Check sheet for the modelled part. Datum: model origin and axes. Units: mm. Give positions to 0.01 mm unless a question says otherwise; leave off trailing zeros. Order: outer loops, then holes, each group sorted by start corner. A loop starts at its lowest first (then second) coordinate and runs counter-clockwise, first axis right, second up.
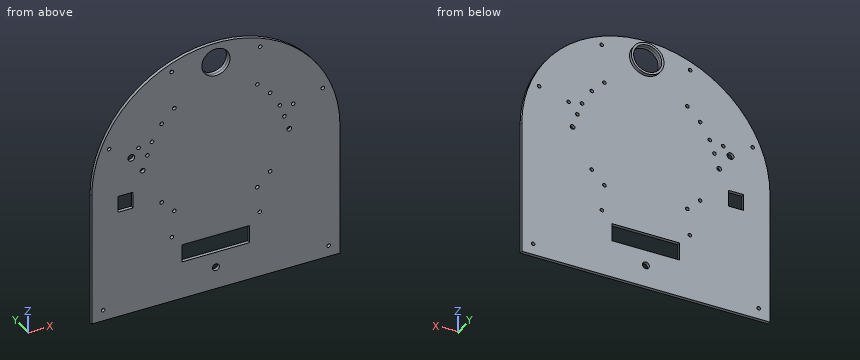
```python
from build123d import *

# Parameters (mm, degrees)
EXTRUDE_START            = -1
EXTRUDE_1_DEPTH          = 3
SKETCH_2_R               = 12.5
CUT_EXTRUDE_1_DEPTH      = 10
SKETCH_3_W               = 220
SKETCH_3_H               = 40
EXTRUDE_2_DEPTH          = 3
CUT_EXTRUDE_2_DEPTH      = 163.815846895
CUT_EXTRUDE_2_DEPTH_BACK = 163.815846895
SKETCH_4_W               = 60
SKETCH_4_H               = 16
SKETCH_5_R               = 1.6
SKETCH_5_R_2             = 2.1
SKETCH_5_R_3             = 3
SKETCH_5_R_4             = 3.1
SKETCH_5_W               = 13.3
SKETCH_5_H               = 14.8
CUT_EXTRUDE_3_DEPTH      = 10
SKETCH_7_R               = 1.6
CUT_EXTRUDE_6_DEPTH      = 162.347451173
SKETCH_8_R               = 1.6
CUT_EXTRUDE_7_DEPTH      = 162.347451173
SHEET_EXTRUDE_1_1_DEPTH  = 3
THICKEN_1_T2             = 2


with BuildPart() as part:
    # 草图1 → 凸台-拉伸1 (new body)
    with BuildSketch(Plane(origin=(0, 0, 0), x_dir=(1, 0, 0), z_dir=(0, 1, 0)).offset(EXTRUDE_START)):
        with BuildLine():
            Line((-110, 0), (-110, 80))
            Line((-110, 80), (110, 80))
            Line((110, 80), (110, 0))
            ThreePointArc((110, 0), (0, -110), (-110, 0))
        make_face()
    extrude(amount=EXTRUDE_1_DEPTH)

    # 草图2 → 切除-拉伸1 (cut)
    with BuildSketch(Plane(origin=(0, 2, 0), x_dir=(1, 0, 0), z_dir=(0, 1, 0))):
        with Locations(Location((0, -92, 0), (0, 0, 270))):
            Circle(SKETCH_2_R)
    extrude(amount=-CUT_EXTRUDE_1_DEPTH, mode=Mode.SUBTRACT)

    # 草图3 → 凸台-拉伸2 (add)
    with BuildSketch(Plane(origin=(0, 2, 0), x_dir=(1, 0, 0), z_dir=(0, 1, 0))):
        with Locations((0, 100)):
            Rectangle(SKETCH_3_W, SKETCH_3_H)
    extrude(amount=-EXTRUDE_2_DEPTH)

    # 草图4 → 切除-拉伸2 (cut, two sides: drawn at the far end of the back side and taken through both)
    with BuildSketch(Plane(origin=(0, 2, 0), x_dir=(1, 0, 0), z_dir=(0, 1, 0)).offset(-CUT_EXTRUDE_2_DEPTH_BACK)):
        with Locations((0, 78)):
            Rectangle(SKETCH_4_W, SKETCH_4_H)
    extrude(amount=CUT_EXTRUDE_2_DEPTH + CUT_EXTRUDE_2_DEPTH_BACK, mode=Mode.SUBTRACT)

    # 草图5 → 切除-拉伸3 (cut)
    with BuildSketch(Plane(origin=(0, 2, 0), x_dir=(1, 0, 0), z_dir=(0, 1, 0))):
        with Locations(Location((94.697652082, -39.225051817, 0), (0, 0, 270))):
            Circle(SKETCH_5_R)
        with Locations(Location((39.225051817, -94.697652082, 0), (0, 0, 270))):
            Circle(SKETCH_5_R)
        with Locations(Location((-39.225051817, -94.697652082, 0), (0, 0, 270))):
            Circle(SKETCH_5_R)
        with Locations(Location((-94.697652082, -39.225051817, 0), (0, 0, 270))):
            Circle(SKETCH_5_R)
        with Locations(Location((-65, -10, 0), (0, 0, 270))):
            Circle(SKETCH_5_R_2)
        with Locations(Location((65, -10, 0), (0, 0, 270))):
            Circle(SKETCH_5_R_2)
        with Locations(Location((-75, -25, 0), (0, 0, 270))):
            Circle(SKETCH_5_R_3)
        with Locations(Location((-100, 110, 0), (0, 0, 270))):
            Circle(SKETCH_5_R)
        with Locations(Location((100, 110, 0), (0, 0, 270))):
            Circle(SKETCH_5_R)
        with Locations(Location((-39, 60, 0), (0, 0, 270))):
            Circle(SKETCH_5_R)
        with Locations(Location((39, 60, 0), (0, 0, 270))):
            Circle(SKETCH_5_R)
        with Locations(Location((0, 100, 0), (0, 0, 270))):
            Circle(SKETCH_5_R_4)
        with Locations((-80, 15)):
            Rectangle(SKETCH_5_W, SKETCH_5_H)
    extrude(amount=-CUT_EXTRUDE_3_DEPTH, mode=Mode.SUBTRACT)

    # 草图7 → 切除-拉伸6 (cut, through all)
    with BuildSketch(Plane(origin=(0, 2, -2), x_dir=(1, 0, 0), z_dir=(0, -1, 0))):
        with Locations(Location((-48.083261121, -22.769552622, 0), (0, 0, 270))):
            Circle(SKETCH_7_R)
        with Locations(Location((-36.769552622, -34.083261121, 0), (0, 0, 270))):
            Circle(SKETCH_7_R)
        with Locations(Location((48.083261121, -22.769552622, 0), (0, 0, 90))):
            Circle(SKETCH_7_R)
        with Locations(Location((36.769552622, -34.083261121, 0), (0, 0, 90))):
            Circle(SKETCH_7_R)
        with Locations(Location((-48.083261121, 50.769552622, 0), (0, 0, 90))):
            Circle(SKETCH_7_R)
        with Locations(Location((-36.769552622, 62.083261121, 0), (0, 0, 90))):
            Circle(SKETCH_7_R)
        with Locations(Location((36.769552622, 62.083261121, 0), (0, 0, 270))):
            Circle(SKETCH_7_R)
        with Locations(Location((48.083261121, 50.769552622, 0), (0, 0, 270))):
            Circle(SKETCH_7_R)
    extrude(amount=CUT_EXTRUDE_6_DEPTH, mode=Mode.SUBTRACT)

    # 草图8 → 切除-拉伸7 (cut, through all)
    with BuildSketch(Plane(origin=(0, 2, -2), x_dir=(1, 0, 0), z_dir=(0, -1, 0))):
        with Locations(Location((68.577848346, 34.394141003, 0), (0, 0, 270))):
            Circle(SKETCH_8_R)
        with Locations(Location((60.784462756, 25.106345729, 0), (0, 0, 270))):
            Circle(SKETCH_8_R)
        with Locations(Location((56.637688898, 36.499513268, 0), (0, 0, 270))):
            Circle(SKETCH_8_R)
        with Locations(Location((-60.784462756, 25.106345729, 0), (0, 0, 90))):
            Circle(SKETCH_8_R)
        with Locations(Location((-56.637688898, 36.499513268, 0), (0, 0, 90))):
            Circle(SKETCH_8_R)
        with Locations(Location((-68.577848346, 34.394141003, 0), (0, 0, 90))):
            Circle(SKETCH_8_R)
    extrude(amount=CUT_EXTRUDE_7_DEPTH, mode=Mode.SUBTRACT)

    # Sheet 凸台-拉伸1: a surface, the sketch's curves swept straight by 3 mm
    with BuildLine(Plane(origin=(0, 2, 0), x_dir=(1, 0, 0), z_dir=(0, 1, 0)), mode=Mode.PRIVATE) as sheet_extrude_1_1_path:
        CenterArc((0, -92), 12.5, 0, 360)
    sheet_extrude_1_1 = Shell.extrude(sheet_extrude_1_1_path.wire(), (0 * SHEET_EXTRUDE_1_1_DEPTH, 1 * SHEET_EXTRUDE_1_1_DEPTH, 0 * SHEET_EXTRUDE_1_1_DEPTH))
    add(Solid.thicken(sheet_extrude_1_1, -THICKEN_1_T2))


solid = part.part
```
Q1. Material ranges on line 1 (X direction, y = 0.85, z = -21); line 2 (Y direction, x = 28.5, z = 66); line 3 (X direction, y = 0.7, z = -100), recorded low to high.
Q2. Sectioned sample at C-C, the plane x = -84. Record the cut outline in (y, z).
Q3. Sectioned sample at A-A, the plane z = -13. Record the cut outline in (x, y), plus the area to 3 significant figures.
Q4. Go/stop test with flat-tipped pins: P1, Ø2, axis at y = 0.5, z = 42, coming from the -X side; P2, Ø3, axis at x = 68.58, z = 32.39, coming from the -Y side; P3, Ø2.5, axis at x = -82, y = 0.5, coming from the +Z side; P4, Ø1.5, axis at x = 60.5, z = -89, coming from the +Y side. Record where each tip stops, or that it passes through.
Q5. Sectioned sample at D-D, the plane x = 43.5. Record the cut outline in (y, z).
Q6. Sectioned sample at B-B, the plane x = 0. Record the cut outline in (y, z), plus the area to 3 significant figures.
Filled in:
1. line 1: x = -110 to -86.65, -73.35 to 110
1. line 2: y = -1 to 2
1. line 3: x = -110 to -3.1, 3.1 to 110
2. outline: (-1, -120) - (2, -120) - (2, -22.4) - (-1, -22.4) - close; (-1, -7.6) - (2, -7.6) - (2, 71.02) - (-1, 71.02) - close
3. outline: (-110, -1) - (-86.65, -1) - (-86.65, 2) - (-110, 2) - close; (-73.35, -1) - (110, -1) - (110, 2) - (-73.35, 2) - close
3. area: 620 mm2
4. P1: stops at x = -102.07
4. P2: passes through
4. P3: stops at z = 74.7
4. P4: stops at y = 2
5. outline: (-1, -120) - (2, -120) - (2, 101.03) - (-1, 101.03) - close
6. outline: (-1, -120) - (2, -120) - (2, -103.1) - (-1, -103.1) - close; (-1, -96.9) - (2, -96.9) - (2, -86) - (-1, -86) - close; (-1, -70) - (2, -70) - (2, 77.5) - (5, 77.5) - (5, 79.5) - (-1, 79.5) - close; (-1, 104.5) - (5, 104.5) - (5, 106.5) - (2, 106.5) - (2, 110) - (-1, 110) - close
6. area: 560 mm2
